```python
from build123d import *
from OCP.BRepFilletAPI import BRepFilletAPI_MakeChamfer

# Parameters (mm, degrees)
BOSS_EXTRUDE1_DEPTH = 27.432
CHAMFER1_SIZE       = 0.254
CHAMFER1_SIZE2      = 0.146646968


# Read off the part's stored shape, not the designer's step: Cut-Revolve4
with BuildPart() as part:
    # Sketch3 → Boss-Extrude1 (new body)
    with BuildSketch(Plane(origin=(0, 0, 0), x_dir=(1, 0, 0), z_dir=(0, 1, 0))):
        Polygon((4.7625, 2.749630657), (0, 5.499261314), (-4.7625, 2.749630657), (-4.7625, -2.749630657), (0, -5.499261314), (4.7625, -2.749630657), align=None)
    extrude(amount=BOSS_EXTRUDE1_DEPTH)

    # Cut-Revolve4 outline → Cut-Revolve4 (revolve, cut)
    with BuildSketch(Plane.XY):
        Polygon((4.6609, 9.18188181), (3.1369, 8.302), (5.499261314, 8.302), (5.499261314, 27.432), (2.54, 27.432), (2.54, 16.302), (3.1369, 16.302), (4.6609, 15.42211819), align=None)
        Polygon((0.99695, 21.082), (2, 21.082), (2, 27.432), (0, 27.432), (0, 1.391072642), (0.99695, 1.92116036), align=None)
    revolve(axis=Axis((0, 0, 0), (0, 1, 0)), mode=Mode.SUBTRACT)

    # Chamfer1: one chamfer whose edges measure the first distance from different faces: ONE call of the kernel's chamfer builder (chamfer() names one face for all edges)
    chamfer1_edges_1 = [part.edges().sort_by_distance(p)[0] for p in [
        (-2.54, 27.432, 0),
    ]]
    chamfer1_side_1 = [part.faces().sort_by_distance(p)[0] for p in [
        (-2.468157951, 27.432, 0),
    ]]
    chamfer1_edges_2 = [part.edges().sort_by_distance(p)[0] for p in [
        (-2, 27.432, 0),
    ]]
    chamfer1_side_2 = [part.faces().sort_by_distance(p)[0] for p in [
        (-2, 24.257, 0),
    ]]
    chamfer1 = BRepFilletAPI_MakeChamfer(part.part.solid().wrapped)
    for e in chamfer1_edges_1:
        chamfer1.Add(CHAMFER1_SIZE, CHAMFER1_SIZE2, e.wrapped, chamfer1_side_1[0].wrapped)  # the first distance lies on this face
    for e in chamfer1_edges_2:
        chamfer1.Add(CHAMFER1_SIZE, CHAMFER1_SIZE2, e.wrapped, chamfer1_side_2[0].wrapped)  # the first distance lies on this face
    add(Compound.cast(chamfer1.Shape()), mode=Mode.REPLACE)

    # Sketch4 → Cut-Revolve5 (revolve, cut)
    with BuildSketch(Plane.XY, mode=Mode.PRIVATE) as cut_revolve5_sk:
        Polygon((-0.25, 0.762), (-0.5, 0.762), (-3, 2.091273579), (-3, 5.762), (-6.107414125, 5.762), (-6.107414125, 0), (0, 0), (0, 1.524), (-0.25, 1.524), align=None)
    revolve(cut_revolve5_sk.sketch.rotate(Axis((0, 0, 0), (0, 1, 0)), 270), axis=Axis((0, 0, 0), (0, 1, 0)), mode=Mode.SUBTRACT)


solid = part.part
```
The model under review builds one solid part; all positions refer to its coordinate system, in mm. A direction names the side the tool comes from. Give positions to 0.01 mm unless a question says otherwise; leave off trailing zeros. Write each loop counter-clockwise with the first axis right and the second up, starting at its lowest first coordinate (ties: lowest second). Pieces come first, ordered by that corner, then holes.
(1) The part is to be moulded in two halves that separate along Y. For faces 4 (the cylindrical face through (0, 24, 2)), 5 (the flat face through (-2.2, 5.762, 2.4)), 6 (the flat face through (3.24, 8.302, 1.15)), 7 (the flat face through (-1, 21.082, 1)), say which applies: released by +Y, released by -Y, zero draft, split by the parting line, or undercut.
(2) Tool access review of faces 1 (the cylindrical face through (-0.9, 3.95, -2.86)), 2 (the flat face through (2.348, 7.014, 4.144)), 3 (the cylindrical face through (0.95, 11.64, -0.3)): name each direction out of +Z, -Z, +X, -X, +Y, -Y from which nothing blocks a thin tool from reaching the whole face with its end or side.
(3) Consider section B-B, the plane y = 14.25. Give the boundary of the cut face in (x, z).
(4) To check wall thickness, follow L1, parallel to X at y = 10.5, z = 0; L2, parallel to Z at x = 0, y = 23.25. State the ranges of each line that lie inside material, in increasing order.
(5) Consider section C-C, the plane y = 20.75. Give the boundary of the cut face in (x, z), and give its area (3 significant figures).
(6) Consider section A-A, the plane y = 7.5. Give the boundary of the cut face in (x, z).
(7) For P1, Ø1.2, axis at x = 0.5, z = -1, coming from the +Y side; P2, Ø4, axis at y = 10.5, z = -1, coming from the -X side; P3, Ø3, axis at x = -1.5, z = 2.5, coming from the -Y side, all flat-tipped, find the tip position at first contact; note any pin that passes through.
Returned:
1. face 4: zero draft
1. face 5: released by -Y
1. face 6: undercut
1. face 7: released by +Y
2. face 1: -Y
2. face 2: +Z, +X, +Y, -Y
2. face 3: +Y
3. outline: circle Ø9.32 at (0, 0); hole circle Ø1.99 at (0, 0)
4. L1: x = -4.66 to -1, 1 to 4.66
4. L2: z = -2.54 to -2, 2 to 2.54
5. outline: circle Ø5.08 at (0, 0); hole circle Ø1.99 at (0, 0)
5. area: 17.1 mm2
6. outline: (-4.76, -2.75) - (0, -5.5) - (4.76, -2.75) - (4.76, 2.75) - (0, 5.5) - (-4.76, 2.75) - close; hole circle Ø1.99 at (0, 0)
7. P1: stops at y = 21.08
7. P2: stops at x = -4.66
7. P3: stops at y = 1.25
